Autodesk Inventor part; units mm, degrees
ref_plane "YZ Plane" through (0, 0, 0) normal (1, 0, 0) x (0, 1, 0)
ref_plane "XZ Plane" through (0, 0, 0) normal (0, 1, 0) x (-1, 0, 0)
ref_plane "XY Plane" through (0, 0, 0) normal (0, 0, 1) x (1, 0, 0)
sketch "Sketch1" plane through (0, 0, 0) normal (0, 1, 0) x (-1, 0, 0)
  circle A0 centre (0, 0) radius 4
  circle A1 centre (0, 0) radius 6
  dimension "d0" = 8
  dimension "d1" = 2
extrude "Extrusion1" add sketch "Sketch1" along normal blind 4
sketch "Sketch2" plane through (0, 4, 0) normal (0, 1, 0) x (1, 0, 0)
  circle A0 centre (0, 0) radius 12.5
  circle A1 centre (0, 0) radius 4
  dimension "d4" = 25
extrude "Extrusion2" add sketch "Sketch2" along normal blind 3
sketch "Sketch3" plane through (0, 7, 0) normal (0, 1, 0) x (1, 0, 0)
  circle A0 centre (-18.5, 0) radius 2.5
  circle A1 centre (18.5, 0) radius 2.5
  circle A2 centre (0, 0) radius 12.5 construction
  circle A3 centre (0, 0) radius 14.5
  circle A4 centre (-18.5, 0) radius 4.5
  circle A5 centre (18.5, 0) radius 4.5
  line L0 (-20.9324, 3.7859) -> (-7.8378, 12.1991)
  line L1 (-20.9324, -3.7859) -> (-7.8378, -12.1991)
  line L2 (20.9324, 3.7859) -> (7.8378, 12.1991)
  line L3 (20.9324, -3.7859) -> (7.8378, -12.1991)
  circle A6 centre (0, 0) radius 4
  point P0 (-14.3851, -1.8215)
  point P1 (-14.3851, 1.8215)
  point P2 (14.3851, 1.8215)
  point P3 (14.3851, -1.8215)
  dimension "d7" = 5
  dimension "d8" = 5
  dimension "d9" = 37
  dimension "d10" = 18.5
  dimension "d11" = 2
  dimension "d12" = 2
  dimension "d13" = 2
extrude "Extrusion3" add sketch "Sketch3" along normal blind 3
properties part number "screw_bracket"
Read the model definition and answer for the solid it produces. Units are mm, in the model's axes. A direction names the side the tool comes from. Give positions to 0.01 mm unless a question says otherwise; leave off trailing zeros. Write each loop counter-clockwise with the first axis right and the second up, starting at its lowest first coordinate (ties: lowest second). Pieces come first, ordered by that corner, then holes. Notation, with made-up numbers: (-36, -23) -> (-5, -23) arc R27 cw to (-5, 7) -> close; hole circle Ø10 at (20, -25). An arc over 180 degrees is marked (long way). Answer as a JSON object with one key per item and string values. Group by question number.
1) Find section A-A (z = -3.25). Write down the section's boundary in (x, y).
2) Find section C-C (x = 18.5). Write down the section's boundary in (y, z).
3) Find section D-D (y = 8). Write down the section's boundary in (x, z), and give its area (3 significant figures).
4) Each of these flat-tipped pins is pushed along its axis until it touches: P1, Ø5, axis at x = 1, y = 2.5, coming from the -Z side; P2, Ø5, axis at x = -12.5, y = 6, coming from the +Z side; P3, Ø6, axis at x = 16, y = 8.5, coming from the +Z side. Where does it stop, or does it pass through?
5) The mould has two halves that part along Z. Classify faces 1 (the cylindrical face through (0.1, 8.5, 14.5)), 2 (the cylindrical face through (-21, 8, 0)), 3 (the cylindrical face through (11.923, 5.479, 3.755)): +Z half, -Z half, draft (parallel to the pull), parting line (faces both ways), or undercut.
6) Consider L1, parallel to X at y = 8.85, z = 0; L2, parallel to X at y = 5, z = 0; L3, parallel to Z at x = 0, y = 2. Determine where each line is inside the solid, lowest interval first. Write a range as from..to.
7) A tool of negligible diameter and unlimited length cuts with its end or side. For faces 4 (the flat face through (7, 7, 11)), 5 (the flat face through (14.48, 8.48, -7.93)), from which of +Z, -Z, +X, -X, +Y, -Y can it reach the whole face along a straight path? Write none if from no direction.
Values follow:
{
 "1": {"outline": "(-21.61, 7) -> (-12.07, 7) -> (-12.07, 4) -> (-5.04, 4) -> (-5.04, 0) -> (-2.33, 0) -> (-2.33, 10) -> (-21.61, 10) -> close; (2.33, 0) -> (5.04, 0) -> (5.04, 4) -> (12.07, 4) -> (12.07, 7) -> (21.61, 7) -> (21.61, 10) -> (2.33, 10) -> close"},
 "2": {"outline": "(7, -5.35) -> (10, -5.35) -> (10, -2.5) -> (7, -2.5) -> close; (7, 2.5) -> (10, 2.5) -> (10, 5.35) -> (7, 5.35) -> close"},
 "3": {"outline": "(-20.93, -3.79) -> (-7.84, -12.2) arc R14.5 ccw to (7.84, -12.2) -> (20.93, -3.79) arc R4.5 ccw to (20.93, 3.79) -> (7.84, 12.2) arc R14.5 ccw to (-7.84, 12.2) -> (-20.93, 3.79) arc R4.5 ccw to start; hole circle Ø5 at (-18.5, 0); hole circle Ø8 at (0, 0); hole circle Ø5 at (18.5, 0)", "area": "783 mm2"},
 "4": {"P1": "stops at z = -12.5", "P2": "stops at z = 10.68", "P3": "stops at z = 8.88"},
 "5": {"face 1": "+Z half", "face 2": "undercut", "face 3": "parting line"},
 "6": {"L1": "x = -23..-21, -16..-4, 4..16, 21..23", "L2": "x = -12.5..-4, 4..12.5", "L3": "z = -6..-4, 4..6"},
 "7": {"face 4": "-Y", "face 5": "-Z, +X, +Y, -Y"}
}
